Work out the finished part from the listing and answer in its coordinate system (mm). Give positions to 0.01 mm unless a question says otherwise; leave off trailing zeros. Loops run counter-clockwise (first coordinate to the right, second up) from the corner with the lowest first, then second, coordinate; pieces in that order, holes last. Notation, with made-up numbers: (51.5, -23) -> (91.5, -23) arc R26 cw to (91.5, 10) -> close; hole circle Ø5 at (14, 30). An arc over 180 degrees is marked (long way). Answer as CSV lines item,"result". Start each with the question number.
1. Find section C-C, the plane x = 1.05. Give the vertices of the cut face in (y, z), and give its area (3 significant figures).
2. Find the intervals of material crossed by line 1 along Z through (x, y) = (0.8, 16.25); line 2 along X through (y, z) = (9, 1.1); line 3 along X through (y, z) = (17.5, 0.95), in increasing order.
3. Find section B-B, the plane z = -1.05. Give the vertices of the cut face in (x, y), and give its area (3 significant figures).
4. Determine the mould class of faces 1 (the face through (-1.25, 10, 0)), 2 (the face through (0, 10, 1.25)), 3 (the face through (0, 10, -1.25)) for opening direction Z: +Z half, -Z half, draft (parallel to the pull), parting line (faces both ways), or undercut.
5. Find section A-A, the plane y = 16.75. Give the vertices of the cut face in (x, z).
from build123d import *

# Parameters (mm, degrees)
F0_W = 2.5
F0_H = 2.5
F3_R = 0.5


with BuildPart() as f2:
    # F2: sweep along a path in F1
    with BuildLine(Plane.XY) as f2_path:
        Line((0, 0), (0, 20))
    # F0 (on Front) → F2 (sweep)
    with BuildSketch(Plane.XZ):
        Rectangle(F0_W, F0_H)
    sweep(path=f2_path.line)

    # F3
    f3_edges = [f2.edges().sort_by_distance(p)[0] for p in [
        (-1.25, 10, -1.25),
        (-1.25, 10, 1.25),
        (1.25, 10, 1.25),
        (1.25, 10, -1.25),
    ]]
    fillet(f3_edges, radius=F3_R)


solid = f2.part
Resolved:
1,outline,"(0, -1.15) -> (20, -1.15) -> (20, 1.15) -> (0, 1.15) -> close"
1,area,"46.0 mm^2"
2,line 1,"z = -1.25 to 1.25"
2,line 2,"x = -1.11 to 1.11"
2,line 3,"x = -1.21 to 1.21"
3,outline,"(-1.15, 0) -> (1.15, 0) -> (1.15, 20) -> (-1.15, 20) -> close"
3,area,"46.0 mm^2"
4,face 1,"draft"
4,face 2,"+Z half"
4,face 3,"-Z half"
5,outline,"(-1.25, -0.75) arc R0.5 ccw to (-0.75, -1.25) -> (0.75, -1.25) arc R0.5 ccw to (1.25, -0.75) -> (1.25, 0.75) arc R0.5 ccw to (0.75, 1.25) -> (-0.75, 1.25) arc R0.5 ccw to (-1.25, 0.75) -> close"
